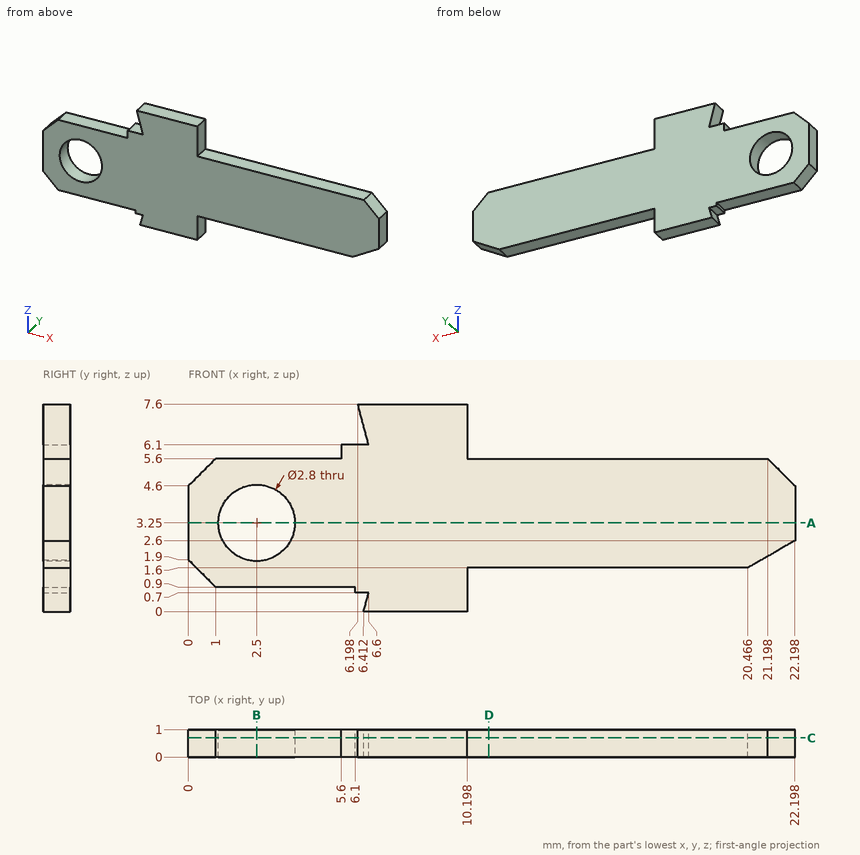
Print and shaded views of the part. All mm, measured from the part's lowest x, y and z. Coordinates: 2 decimals unless noted, no trailing zeros. Order: outer loops, then holes, each group sorted by start corner. A loop starts at its lowest first (then second) coordinate and runs counter-clockwise, first axis right, second up.
Item 1: Saw through at A-A on z = 3.25. List the corners of the cut face in (x, y).
Filled in:
outline: (0, 0) - (1.1, 0) - (1.1, 1) - (0, 1) - close; (3.9, 0) - (22.2, 0) - (22.2, 1) - (3.9, 1) - close
Item 2: Saw through at C-C on y = 0.7. List the corners of the cut face in (x, z).
Filled in:
outline: (0, 1.9) - (1, 0.9) - (6.1, 0.9) - (6.1, 0.7) - (6.6, 0.7) - (6.41, 0) - (10.2, 0) - (10.2, 1.6) - (20.47, 1.6) - (22.2, 2.6) - (22.2, 4.6) - (21.2, 5.6) - (10.2, 5.6) - (10.2, 7.6) - (6.2, 7.6) - (6.6, 6.1) - (5.6, 6.1) - (5.6, 5.6) - (1, 5.6) - (0, 4.6) - close; hole circle Ø2.8 at (2.5, 3.25)
Item 3: Saw through at D-D on x = 11. List the corners of the cut face in (y, z).
Filled in:
outline: (0, 1.6) - (1, 1.6) - (1, 5.6) - (0, 5.6) - close
Item 4: Drill centre lines: L1, parallel to Z at x = 2.5, y = 0.3; L2, parallel to Z at x = 18, y = 0.45; L3, parallel to X at y = 0.4, z = 4.5 (1 decimal). Where is each one in solid material? Low to high.
Filled in:
L1: z = 0.9 to 1.85, 4.65 to 5.6
L2: z = 1.6 to 5.6
L3: x = 0 to 1.9, 3.1 to 22.2
Item 5: Drop flat-ended pins along their axis: pin 1 Ø0.5 at (x, y) = (6, 0.5) entering from +Z; pin 2 Ø0.5 at (y, z) = (0.5, 6.5) entering from +X; pin 3 Ø0.5 at (x, y) = (18, 0.5) entering from +Z. Give the stop position or say it passes through.
Filled in:
pin 1: stops at z = 7.6
pin 2: stops at x = 10.2
pin 3: stops at z = 5.6
Item 6: Saw through at B-B on x = 2.5. List the corners of the cut face in (y, z).
Filled in:
outline: (0, 0.9) - (1, 0.9) - (1, 1.85) - (0, 1.85) - close; (0, 4.65) - (1, 4.65) - (1, 5.6) - (0, 5.6) - close
